Model file for the job. Use its own axes, mm. Coordinates: 2 decimals unless noted, no trailing zeros. Write each loop counter-clockwise with the first axis right and the second up, starting at its lowest first coordinate (ties: lowest second). Pieces come first, ordered by that corner, then holes. Notation, with made-up numbers: M 69,-30 L 117,-30 A22 ccw 117,-2 Z; hole C -4,-24.75 d6. An arc over 180 degrees is marked long. Put each result on its own line as item: value. Start each with the question number.
Q1. Cut at D-D (x = 212.5). Write the cut outline in (y, z).
Q2. Cut at B-B (y = 2.15). Give the number of separate pieces and of enclosed holes in the cut face, then the cut area to 3 significant figures.
Q3. Drop flat-ended pins along their axis: pin 1 (1.5 mm diameter, centred on y = 1.5, z = 83.5, fed in from +X); pin 2 (0.9 mm diameter, centred on x = 30, y = 2, fed in from -Z); pin 3 (1.5 mm diameter, centred on y = 1.5, z = 245.5, fed in from +X). Give the stop position or say it passes through.
Q4. Cut at C-C (x = 143.5). Write the cut outline in (y, z).
Q5. Drill centre lines: line 1 along X through (y, z) = (1.25, 162.5); line 2 along X through (y, z) = (2.2, 121); line 3 along Z through (x, y) = (221, 0.85). Where is each one in solid material? Low to high.
Q6. Cut at A-A (z = 68.5). Write the cut outline in (x, y).
```python
from build123d import *

# Parameters (mm, degrees)
SKETCH1_W           = 3
SKETCH1_H           = 50
SKETCH1_H_2         = 3
BOSS_EXTRUDE1_DEPTH = 3


with BuildPart() as part:
    # Sketch1 → Boss-Extrude1 (new body)
    with BuildSketch(Plane(origin=(0, 0, 0), x_dir=(1, 0, 0), z_dir=(0, 1, 0))):
        Polygon((247, -244), (247, -239), (244, -239), (244, -236), (247, -236), (247, -233), (244, -233), (244, -11), (247, -11), (247, -8), (244, -8), (244, -5), (247, -5), (247, 0), (203, 0), (203, 3), (153, 3), (153, -3), (103, -3), (103, 3), (53, 3), (53, -3), (21, -3), (21, 0), (0, 0), (-3, 0), (-3, -244), (0, -244), (21, -244), (21, -241), (53, -241), (53, -247), (103, -247), (103, -241), (153, -241), (153, -247), (203, -247), (203, -244), align=None)
        with Locations((1.5, -173)):
            Rectangle(SKETCH1_W, SKETCH1_H, mode=Mode.SUBTRACT)
        with Locations((238.5, -6.5)):
            Rectangle(SKETCH1_W, SKETCH1_H_2, mode=Mode.SUBTRACT)
        with Locations((1.5, -71)):
            Rectangle(SKETCH1_W, SKETCH1_H, mode=Mode.SUBTRACT)
        with Locations((238.5, -237.5)):
            Rectangle(SKETCH1_W, SKETCH1_H_2, mode=Mode.SUBTRACT)
    extrude(amount=BOSS_EXTRUDE1_DEPTH)


solid = part.part
```
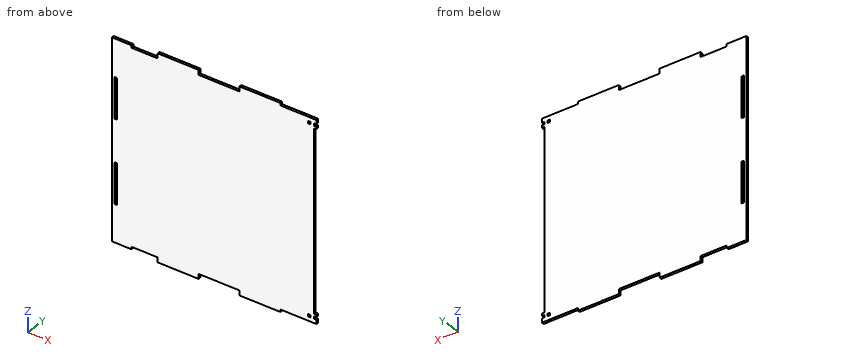
Computed values:
1. outline: M 0,0 L 3,0 L 3,244 L 0,244 Z
2. separate pieces: 1
2. enclosed holes: 4
2. area: 60,100 mm2
3. pin 1: x = 244
3. pin 2: z = 3
3. pin 3: x = 203
4. outline: M 0,3 L 3,3 L 3,241 L 0,241 Z
5. line 1: -3 to 0, 3 to 244
5. line 2: -3 to 244
5. line 3: 0 to 244
6. outline: M -3,0 L 0,0 L 0,3 L -3,3 Z; M 3,0 L 244,0 L 244,3 L 3,3 Z
